from build123d import *

# Parameters (mm, degrees)
EXTRUDE1_DEPTH     = 203.2
SKETCH3_R          = 3.302
CUT_EXTRUDE1_DEPTH = 6.35
SKETCH4_R          = 3.302
CUT_EXTRUDE2_DEPTH = 6.35


with BuildPart() as part:
    # Sketch1 → Extrude1 (new body)
    with BuildSketch(Plane.XY):
        with BuildLine():
            Line((0, 0), (63.5, 0))
            ThreePointArc((63.5, 0), (72.480256121, 3.719743879), (76.2, 12.7))
            Line((76.2, 12.7), (76.2, 158.75))
            ThreePointArc((76.2, 158.75), (79.919743879, 167.730256121), (88.9, 171.45))
            Line((88.9, 171.45), (139.7, 171.45))
            ThreePointArc((139.7, 171.45), (148.680256121, 167.730256121), (152.4, 158.75))
            Line((152.4, 158.75), (152.4, 12.7))
            ThreePointArc((152.4, 12.7), (156.119743879, 3.719743879), (165.1, 0))
            Line((165.1, 0), (228.6, 0))
            Line((228.6, 0), (228.6, 0.133258461))
            Line((228.6, 0.133258461), (228.6, 6.35))
            Line((228.6, 6.35), (171.45, 6.35))
            ThreePointArc((171.45, 6.35), (162.469743879, 10.069743879), (158.75, 19.05))
            Line((158.75, 19.05), (158.75, 165.1))
            ThreePointArc((158.75, 165.1), (155.030256121, 174.080256121), (146.05, 177.8))
            Line((146.05, 177.8), (82.55, 177.8))
            ThreePointArc((82.55, 177.8), (73.569743879, 174.080256121), (69.85, 165.1))
            Line((69.85, 165.1), (69.85, 19.05))
            ThreePointArc((69.85, 19.05), (66.130256121, 10.069743879), (57.15, 6.35))
            Line((57.15, 6.35), (0, 6.35))
            Line((0, 6.35), (0, 0))
        make_face()
    extrude(amount=EXTRUDE1_DEPTH)

    # Sketch3 → Cut-Extrude1 (cut)
    with BuildSketch(Plane(origin=(0, 6.35, 0), x_dir=(-1, 0, 0), z_dir=(0, 1, 0))):
        with Locations((-25.4, 41.275)):
            Circle(SKETCH3_R)
        with Locations((-50.8, 63.5)):
            Circle(SKETCH3_R)
        with Locations((-25.4, 161.925)):
            Circle(SKETCH3_R)
        with Locations((-50.8, 139.7)):
            Circle(SKETCH3_R)
    extrude(amount=-CUT_EXTRUDE1_DEPTH, mode=Mode.SUBTRACT)

    # Sketch4 → Cut-Extrude2 (cut)
    with BuildSketch(Plane(origin=(0, 6.35, 0), x_dir=(-1, 0, 0), z_dir=(0, 1, 0))):
        with Locations((-177.183969253, 74.931336249)):
            Circle(SKETCH4_R)
        with Locations((-177.183969253, 151.131336249)):
            Circle(SKETCH4_R)
        with Locations((-198.01776745, 52.706336249)):
            Circle(SKETCH4_R)
        with Locations((-198.01776745, 173.356336249)):
            Circle(SKETCH4_R)
    extrude(amount=-CUT_EXTRUDE2_DEPTH, mode=Mode.SUBTRACT)


solid = part.part
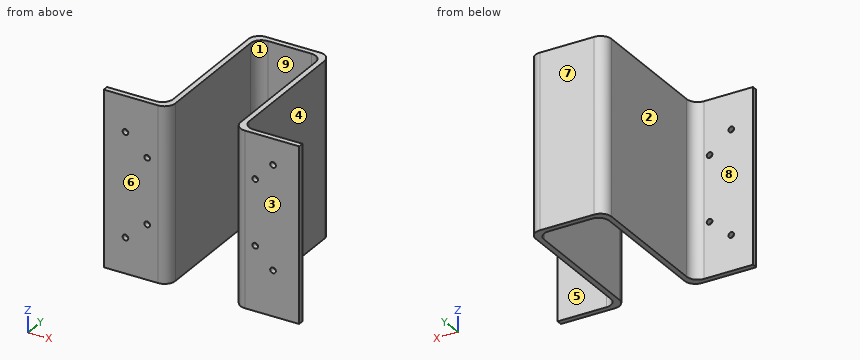
Design review of the part built by this model. Coordinates are the model's own, in mm. Face numbers are marked on the shaded views. A direction names the side the tool comes from. Round coordinates to 2 decimals unless told otherwise and drop trailing zeros. Loops run counter-clockwise (first coordinate to the right, second up) from the corner with the lowest first, then second, coordinate; pieces in that order, holes last. Notation, with made-up numbers: (25.5, -1.5) - (70.5, -1.5) arc R22 cw to (70.5, 33.5) - close; hole circle Ø3 at (10.25, -4). An arc over 180 degrees is marked (long way). One line per question, with ' | ' between items.
1. For the marked faces 5, 6, 7, 8 and 9, list the 3-axis set-ups (+Z, -Z, +X, -X, +Y, -Y) from which the entire face can be reached by the end or side of a thin tool; tool diameter is ignored.
Results are:
face 5: +Z, -Z, +X, +Y | face 6: +Z, -Z, +X, -X, -Y | face 7: +Z, -Z, +X, -X, +Y | face 8: +Z, -Z, -X, +Y | face 9: +Z, -Z, -Y
2. Draft analysis for pull direction X (two halves, no side actions). For the marked faces 1, 2, 3 and 4, state which applies: released by +X, released by -X, zero draft, split by the parting line, or undercut.
Results are:
face 1: undercut | face 2: released by -X | face 3: zero draft | face 4: released by +X
3. Clearance check with flat-ended pins moving along their axes: P1, Ø5.5, axis at x = 50.8, z = 139.7, coming from the +Y side; P2, Ø6, axis at y = 142, z = 117, coming from the +X side; P3, Ø8, axis at x = 142, z = 177.5, coming from the -Y side; P4, Ø7.5, axis at x = 25.4, z = 161.925, coming from the +Y side. State where each tip first meets the part, or that it passes through.
Results are:
P1: passes through | P2: stops at x = 158.75 | P3: stops at y = 169.78 | P4: stops at y = 6.35
4. We need section C-C, the plane z = 139.7. State the section outline as (x, y) points.
Results are:
outline: (0, 0) - (47.5, 0) - (47.5, 6.35) - (0, 6.35) - close; (54.1, 0) - (63.5, 0) arc R12.7 ccw to (76.2, 12.7) - (76.2, 158.75) arc R12.7 cw to (88.9, 171.45) - (139.7, 171.45) arc R12.7 cw to (152.4, 158.75) - (152.4, 12.7) arc R12.7 ccw to (165.1, 0) - (228.6, 0) - (228.6, 6.35) - (171.45, 6.35) arc R12.7 cw to (158.75, 19.05) - (158.75, 165.1) arc R12.7 ccw to (146.05, 177.8) - (82.55, 177.8) arc R12.7 ccw to (69.85, 165.1) - (69.85, 19.05) arc R12.7 cw to (57.15, 6.35) - (54.1, 6.35) - close
5. We need section A-A, the plane x = 25.4. State the section outline as (y, z) points.
Results are:
outline: (0, 0) - (6.35, 0) - (6.35, 37.97) - (0, 37.97) - close; (0, 44.58) - (6.35, 44.58) - (6.35, 158.62) - (0, 158.62) - close; (0, 165.23) - (6.35, 165.23) - (6.35, 203.2) - (0, 203.2) - close
6. For L1, parallel to X at y = 19, z = 31; L2, parallel to Z at x = 25.4, y = 4; L3, parallel to Y at x = 103.5, z = 75, list the stretches that pass through material, from the lowest coordinate up. Write a range as [from, to].
Results are:
L1: x = [69.85, 76.2], [152.4, 158.75] | L2: z = [0, 37.97], [44.58, 158.62], [165.23, 203.2] | L3: y = [171.45, 177.8]
7. We need section D-D, the plane z = 84.5. State the section outline as (x, y) points.
Results are:
outline: (0, 0) - (63.5, 0) arc R12.7 ccw to (76.2, 12.7) - (76.2, 158.75) arc R12.7 cw to (88.9, 171.45) - (139.7, 171.45) arc R12.7 cw to (152.4, 158.75) - (152.4, 12.7) arc R12.7 ccw to (165.1, 0) - (228.6, 0) - (228.6, 6.35) - (171.45, 6.35) arc R12.7 cw to (158.75, 19.05) - (158.75, 165.1) arc R12.7 ccw to (146.05, 177.8) - (82.55, 177.8) arc R12.7 ccw to (69.85, 165.1) - (69.85, 19.05) arc R12.7 cw to (57.15, 6.35) - (0, 6.35) - close
8. We need section B-B, the plane y = 124.5. State the section outline as (x, z) points.
Results are:
outline: (69.85, 0) - (76.2, 0) - (76.2, 203.2) - (69.85, 203.2) - close; (152.4, 0) - (158.75, 0) - (158.75, 203.2) - (152.4, 203.2) - close
